Source: CAD feature listing. Evaluate the final solid. Frame: model axes, mm. A direction names the side the tool comes from. Round coordinates to 2 decimals unless told otherwise and drop trailing zeros. Loops run counter-clockwise (first coordinate to the right, second up) from the corner with the lowest first, then second, coordinate; pieces in that order, holes last. Notation, with made-up numbers: (48, 81.5) -> (82, 81.5) arc R26 cw to (82, 118.5) -> close; hole circle Ø4 at (-39, 44). An arc over 180 degrees is marked (long way). Write item = value, one per line.
Autodesk Inventor part; units mm, degrees
ref_plane "YZ Plane" through (0, 0, 0) normal (1, 0, 0) x (0, 1, 0)
ref_plane "XZ Plane" through (0, 0, 0) normal (0, 1, 0) x (-1, 0, 0)
ref_plane "XY Plane" through (0, 0, 0) normal (0, 0, 1) x (1, 0, 0)
sketch "Sketch1" plane through (0, 0, 0) normal (0, 0, 1) x (1, 0, 0)
  arc A0 (136, 96.5127) -> (109, 107) centre (109, 67) ccw
  line L0 (149, 0) -> (149, 67)
  line L1 (109, 107) -> (89, 107)
  line L2 (149, 0) -> (136, 0)
  line L3 (136, 0) -> (136, 112.2002)
  line L4 (89, 110) -> (109, 110)
  arc A1 (136, 100.4664) -> (109, 110) centre (109, 67) ccw
  line L5 (89, 107) -> (89, 110)
  point P0 (0, 0)
  point P1 (0, 53.5)
  dimension "d0" = 13
  dimension "d1" = 3
extrude "Extrusion1" add sketch "Sketch1" along normal blind 91
sketch "Sketch2" plane through (136, 96.5127, 0) normal (1, 0, 0) x (0, 0, -1)
  line L0 (0, 3.9537) -> (-91, 3.9537)
  line L1 (-87, 3.9537) -> (-4, 3.9537)
  line L2 (-4, 3.9537) -> (-4, -92.0463)
  line L3 (-4, -92.0463) -> (-87, -92.0463)
  line L4 (-87, -92.0463) -> (-87, 3.9537)
  line L5 (-91, 0) -> (-91, 3.9537)
  point P0 (0, -96.5127)
  point P1 (-4, 3.9537)
  dimension "d4" = 83
  dimension "d5" = 96
  dimension "d6" = 4
extrude "Extrusion2" add sketch "Sketch2" against normal blind 3
fillet "Fillet1" radius 8 1 edges at (134.5, 4.4664, 87)
sketch "Sketch3" plane through (136, 96.5127, 0) normal (1, 0, 0) x (0, 0, -1)
  line L0 (-79, -92.0463) -> (-4, -92.0463)
  line L1 (-4, -92.0463) -> (-26, -92.0463)
  line L2 (-26, -92.0463) -> (-26, -7.0463)
  line L3 (-26, -7.0463) -> (-4, -7.0463)
  line L4 (-4, -7.0463) -> (-4, -92.0463)
  point P0 (0, -96.5127)
  dimension "d10" = 22
  dimension "d11" = 85
extrude "Extrusion3" cut sketch "Sketch3" against normal up to surface (3 mm away)
properties part number "obudowa przekładni 3 LEFT"
1. Contact query for flat-ended pins moving along their axis: pin 1 Ø1 at (x, z) = (100.5, 10.5) entering from -Y; pin 2 Ø12 at (y, z) = (58, 74.5) entering from -X; pin 3 Ø3.5 at (x, z) = (135, 11) entering from -Y. Output: stop coordinate, or through.
Evaluation:
pin_1 = 107
pin_2 = 133
pin_3 = 89.47
2. Section query D-D (z = 42). Return the cut outline in (x, y).
Evaluation:
outline = (89, 107) -> (109, 107) arc R40 cw to (133, 99) -> (133, 4.47) -> (136, 4.47) -> (136, 100.47) arc R43 ccw to (109, 110) -> (89, 110) -> close
3. Line query: probe 1 along Y at (x, z) = (96.5, 49); probe 2 along X at (y, z) = (21, 42); probe 3 along Y at (x, z) = (113, 82.5). Output: solid intervals per line, ascending. Write a range as from..to.
Evaluation:
probe_1 = 107..110
probe_2 = 133..136
probe_3 = 106.8..109.81
4. Section query B-B (x = 101). Return the cut outline in (y, z).
Evaluation:
outline = (107, 0) -> (110, 0) -> (110, 91) -> (107, 91) -> close
5. Section query A-A (z = 7). Return the cut outline in (x, y), then the cut area to 3 significant figures.
Evaluation:
outline = (89, 107) -> (109, 107) arc R40 cw to (133, 99) -> (133, 89.47) -> (136, 89.47) -> (136, 100.47) arc R43 ccw to (109, 110) -> (89, 110) -> close
area = 173 mm²
6. Section query C-C (y = 64). Return the cut outline in (x, z).
Evaluation:
outline = (133, 26) -> (136, 26) -> (136, 87) -> (133, 87) -> close
7. Set-up query: faces 1 (the face through (134.479, 6.748, 84.594)), 2 (the face through (135, 89.466, 15)), 3 (the face through (133, 52, 55)). Return all of +Z, -Z, +X, -X, +Y, -Y with unobstructed straight access to the full face (end or side cutting, diameter ignored); none if empty.
Evaluation:
face_1 = +Z, +X, -X, -Y
face_2 = -Z, +X, -X, -Y
face_3 = +Z, -Z, -X, -Y
